Geometry check sheet. Reference: the model listing, model coordinates, mm. A direction names the side the tool comes from. Round coordinates to 2 decimals unless told otherwise and drop trailing zeros. Loops run counter-clockwise (first coordinate to the right, second up) from the corner with the lowest first, then second, coordinate; pieces in that order, holes last.
```python
from build123d import *

# Parameters (mm, degrees)
LINEAR_AUSTRAGEN_D_NN1_DEPTH    = 200
SKIZZE2_R                       = 6
SCHNITT_LINEAR_AUSTRAGEN1_DEPTH = 60


with BuildPart() as part:
    # Skizze1 → Linear-Austragen-Dünn1 (new body)
    with BuildSketch(Plane.XY):
        Polygon((30, 40), (0, 40), (0, -40), (30, -40), (30, -34), (6, -34), (6, 34), (30, 34), align=None)
    extrude(amount=-LINEAR_AUSTRAGEN_D_NN1_DEPTH)

    # Skizze2 → Schnitt-Linear austragen1 (cut)
    with BuildSketch(Plane(origin=(0, 0, 0), x_dir=(1, 0, 0), z_dir=(0, 1, 0))):
        with Locations((14, 50)):
            Circle(SKIZZE2_R)
        with Locations((14, 12)):
            Circle(SKIZZE2_R)
    extrude(amount=-SCHNITT_LINEAR_AUSTRAGEN1_DEPTH, mode=Mode.SUBTRACT)


solid = part.part
```
1) Sectioned sample at A-A, the plane x = 14. Record the cut outline in (y, z), then the cut area to 3 significant figures.
Report:
outline: (-40, -200) - (-34, -200) - (-34, -56) - (-40, -56) - close; (-40, -44) - (-34, -44) - (-34, -18) - (-40, -18) - close; (-40, -6) - (-34, -6) - (-34, 0) - (-40, 0) - close; (34, -200) - (40, -200) - (40, 0) - (34, 0) - close
area: 2,260 mm2
2) Sectioned sample at B-B, the plane z = -12. Record the cut outline in (x, y), then the cut area to 3 significant figures.
Report:
outline: (0, -40) - (8, -40) - (8, -34) - (6, -34) - (6, 34) - (30, 34) - (30, 40) - (0, 40) - close; (20, -40) - (30, -40) - (30, -34) - (20, -34) - close
area: 696 mm2
3) Access from +Z, -Z, +X, -X, +Y, -Y to the whole of each face (thin tool, end or side, straight path). Record for faces 1 (the face through (19.54, -36.96, -47.7)), 2 (the face through (18, 34, -99)), 3 (the face through (15, 40, -99)).
Report:
face 1: -Y
face 2: +Z, -Z, +X
face 3: +Z, -Z, +X, -X, +Y
4) Sectioned sample at D-D, the plane y = 19. Record the cut outline in (x, z).
Report:
outline: (0, -200) - (6, -200) - (6, 0) - (0, 0) - close
5) Sectioned sample at C-C, the plane z = -136. Record the cut outline in (x, y), then the cut area to 3 significant figures.
Report:
outline: (0, -40) - (30, -40) - (30, -34) - (6, -34) - (6, 34) - (30, 34) - (30, 40) - (0, 40) - close
area: 768 mm2
6) Scan lines: line 1 along Z through (x, y) = (14, -36.65); line 2 along X through (y, z) = (-38.25, -12); line 3 along Y through (x, z) = (26, -128). Record each from-to range of solid material in increasing order.
Report:
line 1: z = -200 to -56, -44 to -18, -6 to 0
line 2: x = 0 to 8, 20 to 30
line 3: y = -40 to -34, 34 to 40
7) Mould release check, pull along X, two halves, no side actions. Record for faces 4 (the face through (5, 1, -200)), 5 (the face through (30, -37, -99)), 6 (the face through (19.54, -36.96, -9.7)): +X half, -X half, draft (parallel to the pull), parting line (faces both ways), or undercut.
Report:
face 4: draft
face 5: +X half
face 6: undercut
8) Gauge pin test, flat ends, axial feed: pin 1 (15.5 mm diameter, centred on x = 14, z = -12, fed in from -Y); pin 2 (8 mm diameter, centred on y = 22.5, z = -84, fed in from +X); pin 3 (6 mm diameter, centred on x = 19, y = -30, fed in from +Z) (3 decimals). Record the tip position at first contact, or that the pin passes through.
Report:
pin 1: stops at y = -40
pin 2: stops at x = 6
pin 3: passes through
